from build123d import *

# Parameters (mm, degrees)
SKETCH2_R                = 37.5
BOSS_EXTRUDE1_DEPTH      = 70
BOSS_EXTRUDE2_START      = -30
SKETCH2_3_R              = 12.5
BOSS_EXTRUDE2_DEPTH      = 46.666666667
EXTRUDE_THIN1_DEPTH      = 115
SKETCH5_W                = 100
SKETCH5_H                = 20
SKETCH5_W_2              = 50
BOSS_EXTRUDE3_DEPTH      = 230
CUT_EXTRUDE2_DEPTH       = 298.363414024
CUT_EXTRUDE2_DEPTH_BACK  = 298.363414024
SKETCH5_3_R              = 5
CUT_EXTRUDE1_START       = -30
CUT_EXTRUDE1_OUTLINE_W   = 217.5
CUT_EXTRUDE1_OUTLINE_H   = 230
CUT_EXTRUDE1_OUTLINE_R   = 8.5
CUT_EXTRUDE1_OUTLINE_R_2 = 33.5
CUT_EXTRUDE1_DEPTH       = 100
RIB1_START               = -2.5
RIB1_DEPTH               = 5
FILLET1_R                = 10


# Read off the part's stored shape, not the designer's step: Cut-Extrude1, Rib1
with BuildPart() as part:
    # Sketch2 → Boss-Extrude1 (new body)
    with BuildSketch(Plane(origin=(0, 0, 0), x_dir=(1, 0, 0), z_dir=(0, 1, 0))):
        with Locations(Location((0, 0, 0), (0, 0, 270))):
            Circle(SKETCH2_R)
    extrude(amount=BOSS_EXTRUDE1_DEPTH)



with BuildPart() as body_2:
    # Sketch2<3> → Boss-Extrude2 (new body)
    with BuildSketch(Plane(origin=(0, 0, 0), x_dir=(1, 0, 0), z_dir=(0, 1, 0)).offset(BOSS_EXTRUDE2_START)):
        with Locations(Location((150, 0, 0), (0, 0, 270))):
            Circle(SKETCH2_3_R)
    extrude(amount=BOSS_EXTRUDE2_DEPTH)


with BuildPart() as part_1:
    add(part.part)

    add(body_2.part)  # Extrude-Thin1 merges body 2
    # Sketch3 → Extrude-Thin1 (add, symmetric)
    with BuildSketch(Plane.XY):
        Polygon((-37.5, 0), (74.247392222, 0), (110, -30), (162.5, -30), (162.5, -24), (112.183821406, -24), (76.431213628, 6), (-37.5, 6), align=None)
    extrude(amount=EXTRUDE_THIN1_DEPTH, both=True)

    # Sketch5 → Boss-Extrude3 (add)
    with BuildSketch(Plane.XY.offset(115)):
        with Locations((7.5, 10)):
            Rectangle(SKETCH5_W, SKETCH5_H)
        with Locations((150, -20)):
            Rectangle(SKETCH5_W_2, SKETCH5_H)
    extrude(amount=-BOSS_EXTRUDE3_DEPTH)

    # Sketch5<3> → Cut-Extrude2 (cut, two sides: drawn at the far end of the back side and taken through both)
    with BuildSketch(Plane.XY.offset(115).offset(-CUT_EXTRUDE2_DEPTH_BACK)):
        with Locations((47.5, 10)):
            Circle(SKETCH5_3_R)
        with Locations((135, -20)):
            Circle(SKETCH5_3_R)
    extrude(amount=CUT_EXTRUDE2_DEPTH + CUT_EXTRUDE2_DEPTH_BACK, mode=Mode.SUBTRACT)

    # Cut-Extrude1 outline → Cut-Extrude1 (cut)
    # profile 1 of 3: a face of its own
    with BuildSketch(Plane(origin=(0, 0, 0), x_dir=(1, 0, 0), z_dir=(0, 1, 0)).offset(CUT_EXTRUDE1_START)):
        with Locations((66.25, 0)):
            Rectangle(CUT_EXTRUDE1_OUTLINE_W, CUT_EXTRUDE1_OUTLINE_H)
        with BuildLine():
            ThreePointArc((152.083333333, 12.325166215), (162.5, 0), (152.083333333, -12.325166215))
            Line((152.083333333, -12.325166215), (6.25, -36.975498644))
            ThreePointArc((6.25, -36.975498644), (-37.5, 0), (6.25, 36.975498644))
            Line((6.25, 36.975498644), (152.083333333, 12.325166215))
        make_face(mode=Mode.SUBTRACT)
    # profile 2 of 3: a face of its own
    with BuildSketch(Plane(origin=(0, 0, 0), x_dir=(1, 0, 0), z_dir=(0, 1, 0)).offset(CUT_EXTRUDE1_START)):
        with Locations((150, 0)):
            Circle(CUT_EXTRUDE1_OUTLINE_R)
    # profile 3 of 3: a face of its own
    with BuildSketch(Plane(origin=(0, 0, 0), x_dir=(1, 0, 0), z_dir=(0, 1, 0)).offset(CUT_EXTRUDE1_START)):
        Circle(CUT_EXTRUDE1_OUTLINE_R_2)
    extrude(amount=CUT_EXTRUDE1_DEPTH, mode=Mode.SUBTRACT)

    # Rib1 outline → Rib1 (add)
    with BuildSketch(Plane.XY.offset(RIB1_START)):
        Polygon((139, -10), (139, 16.666666667), (126.985277599, 16.666666667), (63.425085994, 70), (36, 70), (36, 20), (57.5, 20), (57.5, 6), (76.431213628, 6), (112.183821406, -24), (125, -24), (125, -10), align=None)
    extrude(amount=RIB1_DEPTH)

    # Fillet1
    fillet1_edges = [part_1.edges().sort_by_distance(p)[0] for p in [
        (76.431213628, 6, 13.806354192),
        (112.183821406, -24, 10.784707334),
        (110, -30, 0),
        (112.183821406, -24, -10.784707334),
        (125, -10, 9.701542547),
        (76.431213628, 6, -13.806354192),
        (57.5, 20, 15.406333767),
        (126.985277599, 16.666666667, 0),
        (63.425085994, 70, 0),
        (125, -10, -9.701542547),
        (57.5, 20, -15.406333767),
        (74.247392222, 0, 0),
    ]]
    fillet(fillet1_edges, radius=FILLET1_R)


solid = part_1.part
Source: CAD feature listing. Evaluate the final solid. Frame: model axes, mm. A direction names the side the tool comes from. Round coordinates to 2 decimals unless told otherwise and drop trailing zeros. Loops run counter-clockwise (first coordinate to the right, second up) from the corner with the lowest first, then second, coordinate; pieces in that order, holes last. Notation, with made-up numbers: M -20,39.25 L 28,39.25 A18 ccw 28,55.25 Z; hole C 65.5,40 d8. An arc over 180 degrees is marked long. Answer as CSV lines item,"result".
Q1. Cut plane D-D (x = 63). Return the cut outline in (y, z), plus the area to 3 significant figures.
Verdict:
outline,"M 0,-27.38 L 6,-27.38 L 6,-2.5 L 69.47,-2.5 L 69.47,2.5 L 6,2.5 L 6,27.38 L 0,27.38 Z"
area,"646 mm^2"
Q2. Cut plane A-A (z = 0). Return the cut outline in (x, y), plus the area to 3 significant figures.
Verdict:
outline,"M -37.5,0 L -33.5,0 L -33.5,70 L -37.5,70 Z; M 33.5,0 L 70.61,0 A10 cw 77.04,-2.34 L 107.21,-27.66 A10 ccw 113.64,-30 L 141.5,-30 L 141.5,16.67 L 130.62,16.67 A10 cw 124.2,19.01 L 66.21,67.66 A10 ccw 59.79,70 L 33.5,70 Z; M 158.5,-30 L 162.5,-30 L 162.5,16.67 L 158.5,16.67 Z; hole C 47.5,10 d10; hole C 135,-20 d10"
area,"6,880 mm^2"
Q3. Pull-direction query (X, two-part tool) for faces 1 (the face through (74.07, -0.62, 0.37)), 2 (the face through (76.26, 5.38, 13.95)), 3 (the face through (132, -30, 0)), 4 (the face through (63.25, 69.38, 0.04)); classes: +X half, -X half, draft (parallel to the pull), parting line (faces both ways), or undercut.
Verdict:
face 1,"-X half"
face 2,"undercut"
face 3,"draft"
face 4,"+X half"
Q4. Cut plane B-B (x = -2). Return the cut outline in (y, z), plus the area to 3 significant figures.
Verdict:
outline,"M 0,-37.45 L 70,-37.45 L 70,-33.44 L 0,-33.44 Z; M 0,33.44 L 70,33.44 L 70,37.45 L 0,37.45 Z"
area,"561 mm^2"
Q5. Contact query for flat-ended pins moving along their axis: pin 1 (3 mm diameter, centred on x = 118.5, z = 8.5, fed in from +Y); pin 2 (1.2 mm diameter, centred on y = -22, z = 8.5, fed in from -X); pin 3 (10 mm diameter, centred on y = -2, z = -13.5, fed in from +X); pin 4 (6 mm diameter, centred on x = 117.5, z = 23, fed in from +Y). Output: stop coordinate, or through.
Verdict:
pin 1,"stops at y = -24"
pin 2,"stops at x = 99.75"
pin 3,"stops at x = 159.17"
pin 4,"passes through"
Q6. Cut plane C-C (y = 50.5). Return the cut outline in (x, z).
Verdict:
outline,"M 37.42,-2.5 L 86.66,-2.5 L 86.66,2.5 L 37.42,2.5 A37.5 ccw long Z; hole C 0,0 d67"
Q7. Reachability of faces 5 (the face through (128.01, -12.85, 9.6)), 6 (the face through (37, 20, -22)), 7 (the face through (112.449, -23.414, -10.901)), 8 (the face through (29.4, 70, -16.8)), 9 (the face through (43.815, 13.379, -0.433)) from +Z, -Z, +X, -X, +Y, -Y: full face, straight path, thin tool, end or side. Return the list, or none.
Verdict:
face 5,"+Z, +Y"
face 6,"-Z, +X, +Y"
face 7,"-Z, +Y"
face 8,"+Z, -Z, +X, -X, +Y"
face 9,"+Z, -Z"
Q8. Line query: line 1 along Z through (x, y) = (0, 10); line 2 along Y through (x, z) = (135, -0.5); line 3 along X through (y, z) = (-20, 5). Output: solid intervals per line, ascending.
Verdict:
line 1,"z = -37.5 to -33.5, 33.5 to 37.5"
line 2,"y = -30 to -25, -15 to 16.67"
line 3,"x = 98.08 to 107.42, 125 to 130, 140 to 143.13, 156.87 to 161.46"
